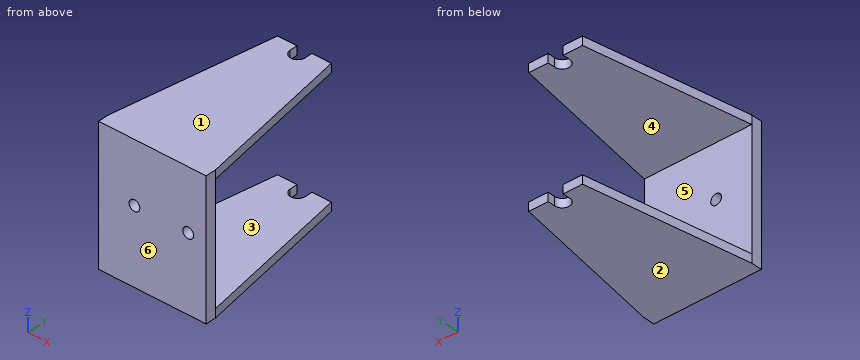
from build123d import *

# Parameters (mm, degrees)
ESTRUSIONE_ESTRUSIONE1_DEPTH = 4
SCHIZZO2_W                   = 50
SCHIZZO2_H                   = 5
ESTRUSIONE_ESTRUSIONE2_DEPTH = 55.13
ESTRUSIONE_ESTRUSIONE3_DEPTH = 4
FORO_PER_VITE_M5_1_D         = 5


with BuildPart() as part:
    # Schizzo1 → Estrusione-Estrusione1 (new body)
    with BuildSketch(Plane.XY):
        with BuildLine():
            Line((-25, 0), (25, 0))
            Line((25, 0), (25, 5))
            Line((25, 5), (12.5, 80))
            Line((12.5, 80), (3.5, 80))
            Line((3.5, 80), (3.5, 76.5))
            ThreePointArc((3.5, 76.5), (0, 73), (-3.5, 76.5))
            Line((-3.5, 76.5), (-3.5, 80))
            Line((-3.5, 80), (-12.5, 80))
            Line((-12.5, 80), (-25, 5))
            Line((-25, 5), (-25, 0))
        make_face()
    extrude(amount=ESTRUSIONE_ESTRUSIONE1_DEPTH)

    # Schizzo2 → Estrusione-Estrusione2 (add)
    with BuildSketch(Plane.XY.offset(4)):
        with Locations((0, 2.5)):
            Rectangle(SCHIZZO2_W, SCHIZZO2_H)
    extrude(amount=ESTRUSIONE_ESTRUSIONE2_DEPTH)

    # Schizzo3 → Estrusione-Estrusione3 (add)
    with BuildSketch(Plane.XY.offset(59.13)):
        with BuildLine():
            Line((3.5, 80), (3.5, 76.5))
            ThreePointArc((3.5, 76.5), (0, 73), (-3.5, 76.5))
            Line((-3.5, 76.5), (-3.5, 80))
            Line((-3.5, 80), (-12.5, 80))
            Line((-12.5, 80), (-25, 5))
            Line((-25, 5), (-25, 0))
            Line((-25, 0), (25, 0))
            Line((25, 0), (25, 5))
            Line((25, 5), (12.5, 80))
            Line((12.5, 80), (3.5, 80))
        make_face()
    extrude(amount=ESTRUSIONE_ESTRUSIONE3_DEPTH)

    # Foro per Vite M5-1 (through all)
    with Locations(Plane(origin=(658.388856913, -5, 71.018331699), x_dir=(-0.2836975166298168, 0, -0.9589138225398959), z_dir=(0, -1, 0))):
        with Locations((223.786948804, -629.129350035), (216.694510888, -605.156504471)):
            Hole(FORO_PER_VITE_M5_1_D / 2)


solid = part.part
Verification items for the finished model (mm, model axes). Face numbers are marked on the shaded views. A direction names the side the tool comes from. Coordinates: 2 decimals unless noted, no trailing zeros. Loops run counter-clockwise (first coordinate to the right, second up) from the corner with the lowest first, then second, coordinate; pieces in that order, holes last. Notation, with made-up numbers: (-14.5, 28) -> (-10.5, 28) arc R24 cw to (-10.5, 66) -> close; hole circle Ø7 at (0, 58). An arc over 180 degrees is marked (long way). Answer as CSV lines item,"result".
1) Cross-section at D-D, the plane z = 33.5. Record the cut outline in (x, y), then the cut area to 3 significant figures.
Found:
outline,"(-25, 0) -> (-10.45, 0) -> (-10.45, 5) -> (-25, 5) -> close; (-6.31, 0) -> (14.55, 0) -> (14.55, 5) -> (-6.31, 5) -> close; (18.69, 0) -> (25, 0) -> (25, 5) -> (18.69, 5) -> close"
area,"209 mm2"
2) Release check for a two-part mould opening along Z. For the marked faces 1, 2, 3 and 4 record: +Z half, -Z half, draft (parallel to the pull), parting line (faces both ways), or undercut.
Found:
face 1,"+Z half"
face 2,"-Z half"
face 3,"undercut"
face 4,"undercut"
3) Cross-section at B-B, the plane y = 74. Record the cut outline in (x, z), then the cut area to 3 significant figures.
Found:
outline,"(-13.5, 0) -> (-2.45, 0) -> (-2.45, 4) -> (-13.5, 4) -> close; (-13.5, 59.13) -> (-2.45, 59.13) -> (-2.45, 63.13) -> (-13.5, 63.13) -> close; (2.45, 0) -> (13.5, 0) -> (13.5, 4) -> (2.45, 4) -> close; (2.45, 59.13) -> (13.5, 59.13) -> (13.5, 63.13) -> (2.45, 63.13) -> close"
area,"177 mm2"
4) Depth check by flat-ended pin: pin 1 (4 mm diameter, centred on y = 79, z = 2, fed in from +X); pin 2 (1 mm diameter, centred on y = 78.5, z = 61.5, fed in from -X); pin 3 (4 mm diameter, centred on y = 77.5, z = 2.5, fed in from -X); pin 4 (4 mm diameter, centred on x = 16.62, z = 34.91, fed in from +Y). Enter the tip coordinate at first touch or a pass-through.
Found:
pin 1,"stops at x = 13"
pin 2,"stops at x = -12.83"
pin 3,"stops at x = -13.25"
pin 4,"passes through"
5) Tool access check on the marked faces 5 and 6. Record the directions out of +Z, -Z, +X, -X, +Y, -Y that give a thin tool (end or side, any length) a straight path to the whole face; none if there is none.
Found:
face 5,"+X, -X, +Y"
face 6,"+Z, -Z, +X, -X, -Y"
6) Thickness scan on L1, parallel to Z at x = -7.5, y = 16; L2, parallel to Y at x = 7.5, z = 10.5. Record the ranges inside material, lowest first. Write a range as from..to.
Found:
L1,"z = 0..4, 59.13..63.13"
L2,"y = 0..5"
7) Cross-section at C-C, the plane x = 0. Record the cut outline in (y, z), then the cut area to 3 significant figures.
Found:
outline,"(0, 0) -> (73, 0) -> (73, 4) -> (5, 4) -> (5, 59.13) -> (73, 59.13) -> (73, 63.13) -> (0, 63.13) -> close"
area,"860 mm2"
8) Cross-section at A-A, the plane y = 23. Record the cut outline in (x, z), then the cut area to 3 significant figures.
Found:
outline,"(-22, 0) -> (22, 0) -> (22, 4) -> (-22, 4) -> close; (-22, 59.13) -> (22, 59.13) -> (22, 63.13) -> (-22, 63.13) -> close"
area,"352 mm2"
